Input: part model. Units: mm. Frame: model coordinates. A direction names the side the tool comes from. Round coordinates to 2 decimals unless told otherwise and drop trailing zeros. Loops run counter-clockwise (first coordinate to the right, second up) from the corner with the lowest first, then second, coordinate; pieces in that order, holes last.
1) Draft query along Y for faces 1 (the face through (19, 26.035, 2)), 2 (the face through (19, 35, 0)), 3 (the face through (19, 57.15, 2)), 4 (the face through (19, 0, 2)). Return one class per face: pulls with the +Y half, pulls with the -Y half, needs draft (parallel to the pull), parting line crosses it, or undercut.
2) Section C-C, the plane z = 2.25. Return loops of the section in (x, y) (3 decimals).
3) Section D-D, the plane y = 28. Return loops of the section in (x, z) (3 decimals).
4) Section B-B, the plane y = 6.35. Return loops of the section in (x, z) (3 decimals), and give its area (3 significant figures).
5) Section A-A, the plane x = 24. Return loops of the section in (y, z) (3 decimals), and give its area (3 significant figures).
6) First-contact query: pin 1 (3 mm diameter, centred on x = 31.75, y = 6.35, fed in from +Z). Flat tip, straight axial feed; report the tip coordinate or a pass-through.
7) Access query for faces 5 (the face through (37.62, 0.46, 1.57)), 6 (the face through (19, 31.115, 2)). Directions: +Z, -Z, +X, -X, +Y, -Y. A direction counts if a zero-diameter tool reaches every point of the face in a straight line with its end or side. Return the directions, or none.
8) Ray query, line 1 along X through (y, z) = (51, 0.9); line 2 along Y through (x, z) = (17, 0.35) (3 decimals); line 3 along Y through (x, z) = (6, 2.8). Return the intervals inside material, ascending.
from build123d import *

# Parameters (mm, degrees)
F0_R     = 1.905
F1_DEPTH = 3.175


with BuildPart() as f1:
    # F0 (on Top) → F1 (new body)
    with BuildSketch(Plane.XY):
        with BuildLine():
            ThreePointArc((0, 1.6002), (0.468688, 0.468688), (1.6002, 0))
            Line((1.6002, 0), (36.4998, 0))
            ThreePointArc((36.4998, 0), (37.631312, 0.468688), (38.1, 1.6002))
            Line((38.1, 1.6002), (38.1, 55.5498))
            ThreePointArc((38.1, 55.5498), (37.631312, 56.681312), (36.4998, 57.15))
            Line((36.4998, 57.15), (1.6002, 57.15))
            ThreePointArc((1.6002, 57.15), (0.468688, 56.681312), (0, 55.5498))
            Line((0, 55.5498), (0, 1.6002))
        make_face()
        with Locations((6.35, 6.35)):
            Circle(F0_R, mode=Mode.SUBTRACT)
        with Locations((31.75, 6.35)):
            Circle(F0_R, mode=Mode.SUBTRACT)
        with Locations((6.35, 50.8)):
            Circle(F0_R, mode=Mode.SUBTRACT)
        with BuildLine():
            ThreePointArc((6.858, 26.035), (4.318, 28.575), (6.858, 31.115))
            Line((6.858, 31.115), (31.242, 31.115))
            ThreePointArc((31.242, 31.115), (33.038051, 30.371051), (33.782, 28.575))
            ThreePointArc((33.782, 28.575), (33.038051, 26.778949), (31.242, 26.035))
            Line((31.242, 26.035), (6.858, 26.035))
        make_face(mode=Mode.SUBTRACT)
        with Locations((31.75, 50.8)):
            Circle(F0_R, mode=Mode.SUBTRACT)
    extrude(amount=F1_DEPTH)


solid = f1.part
Final values:
1. face 1: undercut
1. face 2: needs draft
1. face 3: pulls with the +Y half
1. face 4: pulls with the -Y half
2. outline: (0, 1.6) arc R1.6 ccw to (1.6, 0) - (36.5, 0) arc R1.6 ccw to (38.1, 1.6) - (38.1, 55.55) arc R1.6 ccw to (36.5, 57.15) - (1.6, 57.15) arc R1.6 ccw to (0, 55.55) - close; hole circle Ø3.81 at (6.35, 6.35); hole circle Ø3.81 at (6.35, 50.8); hole (6.858, 26.035) - (31.242, 26.035) arc R2.54 ccw to (33.782, 28.575) arc R2.54 ccw to (31.242, 31.115) - (6.858, 31.115) arc R2.54 ccw to start; hole circle Ø3.81 at (31.75, 6.35); hole circle Ø3.81 at (31.75, 50.8)
3. outline: (0, 0) - (4.384, 0) - (4.384, 3.175) - (0, 3.175) - close; (33.716, 0) - (38.1, 0) - (38.1, 3.175) - (33.716, 3.175) - close
4. outline: (0, 0) - (4.445, 0) - (4.445, 3.175) - (0, 3.175) - close; (8.255, 0) - (29.845, 0) - (29.845, 3.175) - (8.255, 3.175) - close; (33.655, 0) - (38.1, 0) - (38.1, 3.175) - (33.655, 3.175) - close
4. area: 96.8 mm2
5. outline: (0, 0) - (26.035, 0) - (26.035, 3.175) - (0, 3.175) - close; (31.115, 0) - (57.15, 0) - (57.15, 3.175) - (31.115, 3.175) - close
5. area: 165 mm2
6. pin 1: passes through
7. face 5: +Z, -Z, +X, -Y
7. face 6: +Z, -Z
8. line 1: x = 0 to 4.46, 8.24 to 29.86, 33.64 to 38.1
8. line 2: y = 0 to 26.035, 31.115 to 57.15
8. line 3: y = 0 to 4.48, 8.22 to 26.18, 30.97 to 48.93, 52.67 to 57.15
